from build123d import *

# Parameters (mm, degrees)
SKETCH2_W           = 15
SKETCH2_H           = 30
BOSS_EXTRUDE1_DEPTH = 2
SKETCH3_W           = 10
SKETCH3_H           = 5
BOSS_EXTRUDE2_DEPTH = 15
SKETCH4_W           = 6
SKETCH4_H           = 1
CUT_EXTRUDE1_DEPTH  = 15
SKETCH5_W           = 1.25
SKETCH5_H           = 6
SKETCH5_W_2         = 0.75
CUT_EXTRUDE2_DEPTH  = 18.24093965
FILLET1_R           = 5
BOSS_EXTRUDE3_DEPTH = 2
SKETCH7_R           = 0.66453872
BOSS_EXTRUDE4_DEPTH = 5
SKETCH8_W           = 2.454634116
SKETCH8_H           = 5.043768733
BOSS_EXTRUDE5_DEPTH = 2
SKETCH9_R           = 0.923137451
BOSS_EXTRUDE6_DEPTH = 0.5


with BuildPart() as part:
    # Sketch2 → Boss-Extrude1 (new body)
    with BuildSketch(Plane(origin=(0, 0, 0), x_dir=(1, 0, 0), z_dir=(0, 1, 0))):
        Rectangle(SKETCH2_W, SKETCH2_H)
    extrude(amount=BOSS_EXTRUDE1_DEPTH)

    # Sketch3 → Boss-Extrude2 (add)
    with BuildSketch(Plane(origin=(7.5, 0, 0), x_dir=(0, 0, -1), z_dir=(1, 0, 0))):
        with Locations((10, 2.5)):
            Rectangle(SKETCH3_W, SKETCH3_H)
    extrude(amount=-BOSS_EXTRUDE2_DEPTH)

    # Sketch4 → Cut-Extrude1 (cut)
    with BuildSketch(Plane(origin=(7.5, 0, 0), x_dir=(0, 0, -1), z_dir=(1, 0, 0))):
        with Locations((12, 0.5)):
            Rectangle(SKETCH4_W, SKETCH4_H)
        with Locations((12, 2.5)):
            Rectangle(SKETCH4_W, SKETCH4_H)
        with Locations((12, 4.5)):
            Rectangle(SKETCH4_W, SKETCH4_H)
    extrude(amount=-CUT_EXTRUDE1_DEPTH, mode=Mode.SUBTRACT)

    # Sketch5 → Cut-Extrude2 (cut, through all)
    with BuildSketch(Plane(origin=(0, 4, 0), x_dir=(1, 0, 0), z_dir=(0, 1, 0))):
        with Locations((5.625, 12)):
            Rectangle(SKETCH5_W, SKETCH5_H)
        with Locations((2.875, 12)):
            Rectangle(SKETCH5_W, SKETCH5_H)
        with Locations((0.375, 12)):
            Rectangle(SKETCH5_W_2, SKETCH5_H)
        with Locations((-0.375, 12)):
            Rectangle(SKETCH5_W_2, SKETCH5_H)
        with Locations((-2.875, 12)):
            Rectangle(SKETCH5_W, SKETCH5_H)
        with Locations((-5.625, 12)):
            Rectangle(SKETCH5_W, SKETCH5_H)
    extrude(amount=-CUT_EXTRUDE2_DEPTH, mode=Mode.SUBTRACT)

    # Fillet1
    # the kernel refuses this fillet: 5 mm, written as the material it adds along each edge
    with BuildSketch(Plane(origin=(-7.5, 2, -5), x_dir=(0, 1, 0), z_dir=(1, 0, 0))) as fillet1_piece_1:
        with BuildLine():
            CenterArc((5, 4.582575695), FILLET1_R, 180, 66.421821522)
            Line((0, 4.582575695), (-0.1, 4.582575695))
            Line((-0.1, 4.582575695), (-0.1, 0))
            Line((-0.1, 0), (0, -0.1))
            ThreePointArc((0, -0.1), (1.5, -0.1), (2.96, -0.091651514))
            Line((2.96, -0.091651514), (3, 0))
        make_face()
    extrude(amount=15)

    # Sketch6 → Boss-Extrude3 (add)
    with BuildSketch(Plane(origin=(0, 2, 0), x_dir=(1, 0, 0), z_dir=(0, 1, 0))):
        with BuildLine():
            Line((5.106120026, -14.369842053), (5.106120026, -15))
            Line((5.106120026, -15), (6.435197466, -15))
            Line((6.435197466, -15), (6.435197466, -14.369842053))
            ThreePointArc((6.435197466, -14.369842053), (6.472638981, -14.102943479), (6.600769462, -13.865837393))
            ThreePointArc((6.600769462, -13.865837393), (5.770658746, -12.141497566), (4.940548031, -13.865837393))
            ThreePointArc((4.940548031, -13.865837393), (5.068678511, -14.102943479), (5.106120026, -14.369842053))
        make_face()
        with BuildLine():
            Line((-6.435197466, -15), (-6.435197466, -14.369842053))
            ThreePointArc((-6.435197466, -14.369842053), (-6.472638981, -14.102943479), (-6.600769462, -13.865837393))
            ThreePointArc((-6.600769462, -13.865837393), (-5.770658746, -12.141497566), (-4.940548031, -13.865837393))
            ThreePointArc((-4.940548031, -13.865837393), (-5.068678511, -14.102943479), (-5.106120026, -14.369842053))
            Line((-5.106120026, -14.369842053), (-5.106120026, -15))
            Line((-5.106120026, -15), (-6.435197466, -15))
        make_face()
    extrude(amount=BOSS_EXTRUDE3_DEPTH)

    # Sketch7 → Boss-Extrude4 (add)
    with BuildSketch(Plane.XY.offset(15)):
        with Locations((-5.770658746, 3)):
            Circle(SKETCH7_R)
        with Locations((5.770658746, 3)):
            Circle(SKETCH7_R)
    extrude(amount=BOSS_EXTRUDE4_DEPTH)

    # Sketch8 → Boss-Extrude5 (add)
    with BuildSketch(Plane(origin=(0, 2, 0), x_dir=(1, 0, 0), z_dir=(0, 1, 0))):
        with Locations((-5.659720594, -8.745923689)):
            Rectangle(SKETCH8_W, SKETCH8_H)
    extrude(amount=BOSS_EXTRUDE5_DEPTH)

    # Sketch9 → Boss-Extrude6 (add)
    with BuildSketch(Plane(origin=(0, 4, 0), x_dir=(1, 0, 0), z_dir=(0, 1, 0))):
        with Locations(Location((-5.659720594, -8.745923689, 0), (0, 0, 270))):
            Circle(SKETCH9_R)
    extrude(amount=BOSS_EXTRUDE6_DEPTH)


solid = part.part
Geometry check sheet. Reference: the model listing, model coordinates, mm. A direction names the side the tool comes from. Give positions to 0.01 mm unless a question says otherwise; leave off trailing zeros. Order: outer loops, then holes, each group sorted by start corner. A loop starts at its lowest first (then second) coordinate and runs counter-clockwise, first axis right, second up.
1. Draft check along X on faces 1 (the face through (2.25, 1.5, -12)), 2 (the face through (-7, 3, -12)). Enter one of: pulls with the +X half, pulls with the -X half, needs draft (parallel to the pull), parting line crosses it, or undercut.
Completed:
face 1: undercut
face 2: needs draft
2. Access from +Z, -Z, +X, -X, +Y, -Y to the whole of each face (thin tool, end or side, straight path). Record for faces 3 (the face through (4, 4, -12)), 4 (the face through (5.68, 3.66, 17.46)), 5 (the face through (2, 1, -12)), 6 (the face through (-0.75, 3.5, -12)), 7 (the face through (4, 3, -12)).
Completed:
face 3: -Z, +X, -X, +Y
face 4: +Z
face 5: -Z, +X, -X, -Y
face 6: -Z, +Y, -Y
face 7: -Z, +X, -X
3. Sectioned sample at A-A (x = 0). Record the boundary of the cut face in (y, z).
Completed:
outline: (0, -9) - (5, -9) - (5, -5) arc R5 cw to (2, -0.42) - (2, 15) - (0, 15) - close
4. Scan lines: line 1 (X direction, y = 1.2, z = -10); line 2 (X direction, y = 3.5, z = 8); line 3 (Z direction, x = -2, y = 1.1). Record each from-to range of solid material in increasing order.
Completed:
line 1: x = -7.5 to -6.25, -5 to -3.5, -2.25 to -0.75, 0.75 to 2.25, 3.5 to 5, 6.25 to 7.5
line 2: x = -6.89 to -4.43
line 3: z = -15 to 15
5. Depth check by flat-ended pin: pin 1 (1.6 mm diameter, centred on x = -1.5, z = -13.5, fed in from -Y); pin 2 (1 mm diameter, centred on x = -7, z = -11, fed in from +Y); pin 3 (0.7 mm diameter, centred on y = 3, z = 15, fed in from -X). Enter the tip coordinate at first touch or a pass-through.
Completed:
pin 1: stops at y = 1
pin 2: stops at y = 4
pin 3: stops at x = -6.44
6. Sectioned sample at C-C (z = -3). Record the boundary of the cut face in (x, y), then the cut area to 3 significant figures.
Completed:
outline: (-7.5, 0) - (7.5, 0) - (7.5, 2.72) - (-7.5, 2.72) - close
area: 40.8 mm2
7. Sectioned sample at B-B (z = 1.5). Record the boundary of the cut face in (x, y), then the cut area to 3 significant figures.
Completed:
outline: (-7.5, 0) - (7.5, 0) - (7.5, 2) - (-7.5, 2) - close
area: 30.0 mm2
